from build123d import *

# Parameters (mm, degrees)
SKETCH005_R          = 9.525
SKETCH005_R_2        = 4
PAD001_DEPTH         = 0.75
POCKET001_DEPTH      = 54.715989
POCKET001_DEPTH_BACK = 54.715989
POLARPATTERN_COUNT   = 3
SKETCH007_R          = 0.5


with BuildPart() as part:
    # Sketch005 → Pad001 (new body, symmetric)
    with BuildSketch(Plane.XZ):
        Circle(SKETCH005_R)
        Circle(SKETCH005_R_2, mode=Mode.SUBTRACT)
    extrude(amount=PAD001_DEPTH, both=True)

    # Sketch006 → Pocket001 (cut, two sides)
    with BuildSketch(Plane.XZ) as pocket001_sk:
        with BuildLine():
            ThreePointArc((3.25, 5.629165), (0, 6.5), (-3.25, 5.629165))
            Line((-4.7625, 8.248892), (-3.25, 5.629165))
            ThreePointArc((4.7625, 8.248892), (0, 9.525), (-4.7625, 8.248892))
            Line((4.7625, 8.248892), (3.25, 5.629165))
        make_face()
    pocket001 = extrude(amount=-POCKET001_DEPTH, mode=Mode.SUBTRACT) + extrude(pocket001_sk.sketch, amount=POCKET001_DEPTH_BACK, mode=Mode.SUBTRACT)

    # PolarPattern: Pocket001 ×3 about axis
    polarpattern_axis = Axis((0, 0, 0), (0, -1, 0))
    for i in range(1, POLARPATTERN_COUNT):
        add(pocket001.rotate(polarpattern_axis, i * 360 / POLARPATTERN_COUNT), mode=Mode.SUBTRACT)

    # Sketch007 → Groove001 (revolve, cut)
    with BuildSketch(Plane.YZ):
        with Locations((0, 9.7)):
            Circle(SKETCH007_R)
    revolve(axis=Axis((0, 0, 0), (0, 1, 0)), mode=Mode.SUBTRACT)


solid = part.part
Can you work these out from the model? Positions are in its coordinate system, mm. A direction names the side the tool comes from. Give positions to 0.01 mm unless a question says otherwise; leave off trailing zeros. Loops run counter-clockwise (first coordinate to the right, second up) from the corner with the lowest first, then second, coordinate; pieces in that order, holes last. Notation, with made-up numbers: (7.5, -15.75) - (29.5, -15.75) arc R7 ccw to (29.5, -3.75) - close; hole circle Ø7 at (54, 65.25). An arc over 180 degrees is marked (long way). Return JSON: item names as keys, results as strings.
1. If I drill on line 1 (X direction, y = 0.55, z = 6); line 2 (Z direction, x = 0, y = 0.05); line 3 (Z direction, x = -1.25, y = 0.1), over which ranges is the centre line in solid material (lowest first)?
Output values:
{"line 1": "x = -7.4 to -3.46, -2.5 to 2.5, 3.46 to 7.4", "line 2": "z = -9.2 to -4, 4 to 6.5", "line 3": "z = -9.12 to -3.8, 3.8 to 6.38"}
2. For faces 1 (the face through (-5.65, -0.01, -3.21)), 2 (the face through (4.02, -0.01, -6.96)), 3 (the face through (8, 0, 0)), 4 (the face through (-4.02, -0.01, 6.96)), which set-ups out of +Z, -Z, +X, -X, +Y, -Y let a thin tool reach every point of the face, with its end or its side?
Output values:
{"face 1": "-X, +Y, -Y", "face 2": "+X, +Y, -Y", "face 3": "-Z, +X, +Y, -Y", "face 4": "+Z, +Y, -Y"}
3. I want a section at A-A on x = 0. Please give me the cut outline in (y, z) (3 decimals).
Output values:
{"outline": "(-0.75, -9.525) - (-0.468, -9.525) arc R0.5 cw to (0.468, -9.525) - (0.75, -9.525) - (0.75, -4) - (-0.75, -4) - close; (-0.75, 4) - (0.75, 4) - (0.75, 6.5) - (-0.75, 6.5) - close"}
4. I want a section at D-D on z = -6.75. Please give me the cut outline in (x, y), and give its area (3 significant figures).
Output values:
{"outline": "(-3.9, -0.75) - (3.9, -0.75) - (3.9, 0.75) - (-3.9, 0.75) - close", "area": "11.7 mm²"}
5. I want a section at B-B on z = -3. Please give me the cut outline in (x, y), and give its area (3 significant figures).
Output values:
{"outline": "(-5.77, -0.75) - (-2.65, -0.75) - (-2.65, 0.75) - (-5.77, 0.75) - close; (2.65, -0.75) - (5.77, -0.75) - (5.77, 0.75) - (2.65, 0.75) - close", "area": "9.36 mm²"}
6. I'm going to push flat-ended pins straight in: pin 1 Ø3 at (x, z) = (0.5, 0) entering from +Y; pin 2 Ø6 at (x, z) = (-4, -5.5) entering from -Y; pin 3 Ø0.5 at (x, y) = (-8, 0) entering from -Z. Where does each tip first touch, or does it pass through?
Output values:
{"pin 1": "passes through", "pin 2": "stops at y = -0.75", "pin 3": "stops at z = 0"}
7. I want a section at C-C on y = 0.05. Please give me the cut outline in (x, z).
Output values:
{"outline": "(-9.2, 0) - (-6.5, 0) arc R6.5 ccw to (-3.25, -5.63) - (-4.6, -7.97) arc R9.2 ccw to (4.6, -7.97) - (3.25, -5.63) arc R6.5 ccw to (6.5, 0) - (9.2, 0) arc R9.2 ccw to (4.6, 7.97) - (3.25, 5.63) arc R6.5 ccw to (-3.25, 5.63) - (-4.6, 7.97) arc R9.2 ccw to start; hole circle Ø8 at (0, 0)"}
8. We'd pull the mould along X, two halves only. Please class faces 5 (the face through (0, 0, 6.5)), 6 (the face through (-4.02, -0.01, -6.96)), 7 (the face through (-8, 0, 0)), 8 (the face through (-0.867, 0.01, -3.905)): +X half, -X half, draft (parallel to the pull), parting line (faces both ways), or undercut.
Output values:
{"face 5": "undercut", "face 6": "-X half", "face 7": "draft", "face 8": "undercut"}
